For this review, take the finished solid that the model builds, in its own axes (mm). A direction names the side the tool comes from. Give positions to 0.01 mm unless a question says otherwise; leave off trailing zeros. Write item = value, one per line.
```python
from build123d import *

# Parameters (mm, degrees)
F0_W          = 3
F0_H          = 13
F1_DEPTH      = 13.5
F2_W          = 16
F2_H          = 19.6
F3_DEPTH      = 1
F6_DEPTH      = 5000
F7_R          = 2.75
F8_DEPTH      = 50
F9_F1_R       = 3
F9_F2_R       = 3
F9_F3_R       = 3
F9_F4_R       = 2.9999
F10_T1_DEPTH  = 15.0673355609
F10_T3_DEPTH  = 15.0673355609
F10_T5_DEPTH  = 41.7748308216
F10_T7_DEPTH  = 41.7748308216
F10_T9_DEPTH  = 43.4696886285
F10_T11_DEPTH = 12.8188920975
F10_T13_DEPTH = 12.8188920975
F10_T15_DEPTH = 43.4696886285
F10_T17_DEPTH = 33.2132034356
F10_T22_DEPTH = 8.2514565366
F10_S23_R     = 3
F10_T24_DEPTH = 6
F10_T28_DEPTH = 8.2515565366
F10_S29_R     = 3
F10_T30_DEPTH = 6
F10_T34_DEPTH = 10.4999
F10_S35_R     = 3
F10_T36_DEPTH = 7
F10_T40_DEPTH = 10.5
F10_S41_R     = 3
F10_T42_DEPTH = 7


# Not quite as in the source:
# - a fillet or chamfer that OpenCascade refuses, or shapes differently, is made with other operations: its cross-section is extruded or revolved along the edge and cut away or added
# - a fillet or chamfer is up to 0.001 mm smaller than in the source, because OpenCascade refuses the exact size
# - a feature names something its author has since deleted; it is built from what else it names


with BuildPart() as f1:
    # F0 (on Front) → F1 (new body, symmetric)
    with BuildSketch(Plane.XZ):
        with Locations((-1.5, -25.4326644391)):
            Rectangle(F0_W, F0_H)
        Polygon((-10.5673355609, -16.9326644391), (-27.5, 0), (-27.5, 3.3434056677), (-27.5, 25), (-29.5, 25), (-29.5, 0), (-10.5673355609, -18.9326644391), (-3, -18.9326644391), (0, -18.9326644391), (0, -16.9326644391), align=None)
    extrude(amount=F1_DEPTH, both=True)

    # F2 (on face) → F3 (join)
    with BuildSketch(Plane.YZ.offset(-27.5)):
        with Locations((0, 15.2)):
            Rectangle(F2_W, F2_H)
    extrude(amount=F3_DEPTH)

    # F4: F1 across plane


with BuildPart() as f1_1:
    add(f1.part)
    add(f1.part.mirror(Plane.YZ))

    # F5 (on face) → F6 (cut, symmetric)
    with BuildSketch(Plane(origin=(-29.5, 0, 0), x_dir=(0, -1, 0), z_dir=(-1, 0, 0))):
        Polygon((-13.5, 0), (-21.2256871164, 0), (-25.0640398382, -39.3923101205), (-6.5540728933, -39.3923101205), (0.180805733, -37.5877048314), align=None)
    extrude(amount=F6_DEPTH, both=True, mode=Mode.SUBTRACT)

    # F7 (on face) → F8 (cut, symmetric)
    with BuildSketch(Plane.YZ.offset(3)):
        with Locations((-4.9499999732, -25.3868680447)):
            Circle(F7_R)
    extrude(amount=F8_DEPTH, both=True, mode=Mode.SUBTRACT)

    # F9: fillet of radius 3 on 4 edges, made by hand

    # F9_f1
    f9_f1_edges = [f1_1.edges().sort_by_distance(p)[0] for p in [
        (0, 1.8774606434, -31.9326644391),
    ]]
    fillet(f9_f1_edges, radius=F9_F1_R)

    # F9_f2
    f9_f2_edges = [f1_1.edges().sort_by_distance(p)[0] for p in [
        (0, -13.5, -31.9326644391),
    ]]
    fillet(f9_f2_edges, radius=F9_F2_R)

    # F9_f3
    f9_f3_edges = [f1_1.edges().sort_by_distance(p)[0] for p in [
        (3, -5.3615809856, -31.9326644391),
    ]]
    fillet(f9_f3_edges, radius=F9_F3_R)

    # F9_f4 (radius 3 in the source; OpenCascade refuses exactly that, so slightly less here)
    f9_f4_edges = [f1_1.edges().sort_by_distance(p)[0] for p in [
        (-3, -5.3615809856, -31.9326644391),
    ]]
    fillet(f9_f4_edges, radius=F9_F4_R)

    # F10: fillet of radius 3 on 12 edges, made by hand

    # F10_s2 → F10_t1 (cut)
    with BuildSketch(Plane.YZ.offset(3)):
        with BuildLine():
            ThreePointArc((-13.5, -15.9326644391), (-12.6213203436, -18.0539847826), (-10.5, -18.9326644391))
            Line((-10.5, -18.9326644391), (-13.5, -18.9326644391))
            Line((-13.5, -18.9326644391), (-13.5, -15.9326644391))
        make_face()
    extrude(amount=F10_T1_DEPTH, mode=Mode.SUBTRACT)

    # F10_s4 → F10_t3 (cut)
    with BuildSketch(Plane.YZ.offset(-18.0673355609)):
        with BuildLine():
            ThreePointArc((-13.5, -15.9326644391), (-12.6213203436, -18.0539847826), (-10.5, -18.9326644391))
            Line((-10.5, -18.9326644391), (-13.5, -18.9326644391))
            Line((-13.5, -18.9326644391), (-13.5, -15.9326644391))
        make_face()
    extrude(amount=F10_T3_DEPTH, mode=Mode.SUBTRACT)

    # F10_s6 → F10_t5 (cut)
    with BuildSketch(Plane(origin=(-20.0533008589, 0, 20.0533008589), x_dir=(0, 1, 0), z_dir=(0.7071067812, 0, -0.7071067812))):
        with BuildLine():
            ThreePointArc((-13.5, -17.859650045), (-12.6213203436, -19.9809703886), (-10.5, -20.859650045))
            Line((-10.5, -20.859650045), (-13.5, -20.859650045))
            Line((-13.5, -20.859650045), (-13.5, -17.859650045))
        make_face()
    extrude(amount=F10_T5_DEPTH, mode=Mode.SUBTRACT)

    # F10_s8 → F10_t7 (cut)
    with BuildSketch(Plane(origin=(20.0533008589, 0, 20.0533008589), x_dir=(0, 1, 0), z_dir=(-0.7071067812, 0, -0.7071067812))):
        with BuildLine():
            ThreePointArc((-13.5, 17.859650045), (-12.6213203436, 19.9809703886), (-10.5, 20.859650045))
            Line((-10.5, 20.859650045), (-13.5, 20.859650045))
            Line((-13.5, 20.859650045), (-13.5, 17.859650045))
        make_face()
    extrude(amount=F10_T7_DEPTH, mode=Mode.SUBTRACT)

    # F10_s10 → F10_t9 (cut)
    with BuildSketch(Plane(origin=(-6.8077517267, -2.4778189908, -6.8077517267), x_dir=(-0.3420201433, 0.9396926208, 0), z_dir=(0.6847910788, 0.2492435694, 0.6847910788))):
        with BuildLine():
            ThreePointArc((0.3217904404, -21.5780178201), (2.267861443, -21.4075638122), (3.6963913931, -20.0750664959))
            Line((3.6963913931, -20.0750664959), (2.5962561525, -22.1449137726))
            Line((2.5962561525, -22.1449137726), (0.3217904404, -21.5780178201))
        make_face()
    extrude(amount=F10_T9_DEPTH, mode=Mode.SUBTRACT)

    # F10_s12 → F10_t11 (cut)
    with BuildSketch(Plane.YZ.offset(3)):
        with BuildLine():
            ThreePointArc((4.5084510742, -18.9326644391), (6.2291803832, -18.3901205719), (7.3275289366, -16.9587248691))
            Line((7.3275289366, -16.9587248691), (6.6090736888, -18.9326644391))
            Line((6.6090736888, -18.9326644391), (4.5084510742, -18.9326644391))
        make_face()
    extrude(amount=F10_T11_DEPTH, mode=Mode.SUBTRACT)

    # F10_s14 → F10_t13 (cut)
    with BuildSketch(Plane.YZ.offset(-15.8188920975)):
        with BuildLine():
            ThreePointArc((4.5084510742, -18.9326644391), (6.2291803832, -18.3901205719), (7.3275289366, -16.9587248691))
            Line((7.3275289366, -16.9587248691), (6.6090736888, -18.9326644391))
            Line((6.6090736888, -18.9326644391), (4.5084510742, -18.9326644391))
        make_face()
    extrude(amount=F10_T13_DEPTH, mode=Mode.SUBTRACT)

    # F10_s16 → F10_t15 (cut)
    with BuildSketch(Plane(origin=(6.8077517267, -2.4778189908, -6.8077517267), x_dir=(-0.3420201433, -0.9396926208, 0), z_dir=(-0.6847910788, 0.2492435694, 0.6847910788))):
        with BuildLine():
            ThreePointArc((-0.3217904404, -21.5780178201), (-2.267861443, -21.4075638122), (-3.6963913931, -20.0750664959))
            Line((-3.6963913931, -20.0750664959), (-2.5962561525, -22.1449137726))
            Line((-2.5962561525, -22.1449137726), (-0.3217904404, -21.5780178201))
        make_face()
    extrude(amount=F10_T15_DEPTH, mode=Mode.SUBTRACT)

    # F10_s18 → F10_t17 (cut)
    with BuildSketch(Plane.XZ.offset(-16.6066017178)):
        with BuildLine():
            ThreePointArc((28.6213203436, -0.8786796564), (29.2716385975, 0.09459039), (29.5, 1.2426406871))
            Line((29.5, 1.2426406871), (29.5, 0))
            Line((29.5, 0), (28.6213203436, -0.8786796564))
        make_face()
        with BuildLine():
            ThreePointArc((-28.6213203436, -0.8786796564), (-29.2716385975, 0.09459039), (-29.5, 1.2426406871))
            Line((-29.5, 1.2426406871), (-29.5, 0))
            Line((-29.5, 0), (-28.6213203436, -0.8786796564))
        make_face()
    extrude(amount=F10_T17_DEPTH, mode=Mode.SUBTRACT)


with BuildPart() as f10_tool20:
    # F10_s21 → F10_t22 (new body)
    with BuildSketch(Plane.YZ.offset(-3)):
        with BuildLine():
            ThreePointArc((4.5084510742, -18.9326644391), (6.2291803832, -18.3901205719), (7.3275289366, -16.9587248691))
            Line((7.3275289366, -16.9587248691), (6.6090736888, -18.9326644391))
            Line((6.6090736888, -18.9326644391), (4.5084510742, -18.9326644391))
        make_face()
    extrude(amount=F10_T22_DEPTH)

    # F10_s23 → F10_t24 (cut, symmetric)
    with BuildSketch(Plane(origin=(0, -5.0618981212, -13.9074507876), x_dir=(1, 0, 0), z_dir=(0, 0.3420201433, 0.9396926208))):
        with Locations((0, 9.6858503806)):
            Circle(F10_S23_R)
    extrude(amount=F10_T24_DEPTH, both=True, mode=Mode.SUBTRACT)


with BuildPart() as f1_2:
    add(f1_1.part)

    # F10_t19: cut F10_tool20
    add(f10_tool20.part, mode=Mode.SUBTRACT)


with BuildPart() as f10_tool26:
    # F10_s27 → F10_t28 (new body)
    with BuildSketch(Plane.YZ.offset(3)):
        with BuildLine():
            ThreePointArc((4.5084510742, -18.9326644391), (6.2291803832, -18.3901205719), (7.3275289366, -16.9587248691))
            Line((7.3275289366, -16.9587248691), (6.6090736888, -18.9326644391))
            Line((6.6090736888, -18.9326644391), (4.5084510742, -18.9326644391))
        make_face()
    extrude(amount=-F10_T28_DEPTH)

    # F10_s29 → F10_t30 (cut, symmetric)
    with BuildSketch(Plane(origin=(0, -5.0618981212, -13.9074507876), x_dir=(1, 0, 0), z_dir=(0, 0.3420201433, 0.9396926208))):
        with Locations((0, 9.6858503806)):
            Circle(F10_S29_R)
    extrude(amount=F10_T30_DEPTH, both=True, mode=Mode.SUBTRACT)


with BuildPart() as f1_3:
    add(f1_2.part)

    # F10_t25: cut F10_tool26
    add(f10_tool26.part, mode=Mode.SUBTRACT)


with BuildPart() as f10_tool32:
    # F10_s33 → F10_t34 (new body)
    with BuildSketch(Plane.YZ.offset(-3)):
        with BuildLine():
            ThreePointArc((-13.5, -15.9326644391), (-12.6213203436, -18.0539847826), (-10.5, -18.9326644391))
            Line((-10.5, -18.9326644391), (-13.5, -18.9326644391))
            Line((-13.5, -18.9326644391), (-13.5, -15.9326644391))
        make_face()
    extrude(amount=F10_T34_DEPTH)

    # F10_s35 → F10_t36 (cut, symmetric)
    with BuildSketch(Plane.XY.offset(-17.4)):
        with Locations((0, -10.5)):
            Circle(F10_S35_R)
    extrude(amount=F10_T36_DEPTH, both=True, mode=Mode.SUBTRACT)


with BuildPart() as f1_4:
    add(f1_3.part)

    # F10_t31: cut F10_tool32
    add(f10_tool32.part, mode=Mode.SUBTRACT)


with BuildPart() as f10_tool38:
    # F10_s39 → F10_t40 (new body)
    with BuildSketch(Plane.YZ.offset(3)):
        with BuildLine():
            ThreePointArc((-13.5, -15.9326644391), (-12.6213203436, -18.0539847826), (-10.5, -18.9326644391))
            Line((-10.5, -18.9326644391), (-13.5, -18.9326644391))
            Line((-13.5, -18.9326644391), (-13.5, -15.9326644391))
        make_face()
    extrude(amount=-F10_T40_DEPTH)

    # F10_s41 → F10_t42 (cut, symmetric)
    with BuildSketch(Plane.XY.offset(-17.4)):
        with Locations((0, -10.5)):
            Circle(F10_S41_R)
    extrude(amount=F10_T42_DEPTH, both=True, mode=Mode.SUBTRACT)


with BuildPart() as f1_5:
    add(f1_4.part)

    # F10_t37: cut F10_tool38
    add(f10_tool38.part, mode=Mode.SUBTRACT)


solid = f1_5.part
```
1. The part is to be moulded in two halves that separate along X. For faces 6 (the face through (26.5, 0, 15)), 7 (the face through (7, -3, -18.933)), 8 (the face through (3, -4, -22)), 9 (the face through (-19.7, -2.4, -9.8)), say which applies: +X half, -X half, draft (parallel to the pull), parting line (faces both ways), or undercut.
Responses:
face_6 = undercut
face_7 = draft
face_8 = +X half
face_9 = -X half
2. Machinability: for faces 1 (the face through (27.5, 0, 4)), 2 (the face through (-5.346, 6.208, -18.405)), 3 (the face through (-5.85, -12.25, -18.37)), 4 (the face through (-26.5, 0, 15)), 5 (the face through (1.88, -12.84, -22.85)), which of the approach directions +Z, -Z, +X, -X, +Y, -Y give a long, thin tool a straight path to every point of the face, cutting with its end or side? Answer none if there is none.
Responses:
face_1 = none
face_2 = -Z, -X, +Y
face_3 = -Z, -X, -Y
face_4 = +Z, +Y, -Y
face_5 = -Z, -Y
3. For line 1 along X through (y, z) = (-10.75, 2.5); line 2 along Z through (x, y) = (-8, -6); line 3 along Z through (x, y) = (-0.2, -4.95), list the stretches that pass through material, from the lowest coordinate up. Write a range as from..to.
Responses:
line_1 = -29.5..-27.5, 27.5..29.5
line_2 = -18.93..-16.93
line_3 = -31.93..-28.14, -22.64..-16.93
4. Insertion check: P1, Ø3, axis at x = 18.5, y = -4.5, coming from the -Z side; P2, Ø6, axis at x = -5, y = -3.5, coming from the -Z side; P3, Ø8, axis at y = -5.5, z = -26, coming from the -X side. Each pin has a flat end and moves straight along its axis. Give the tip position at first contact, or say it passes through.
Responses:
P1 = -12.5
P2 = -31.17
P3 = -3
